The model under review builds one solid part; all positions refer to its coordinate system, in mm. Face numbers are marked on the shaded views. A direction names the side the tool comes from. Round coordinates to 2 decimals unless told otherwise and drop trailing zeros. Order: outer loops, then holes, each group sorted by start corner. A loop starts at its lowest first (then second) coordinate and runs counter-clockwise, first axis right, second up. Notation, with made-up numbers: M 55,47 L 89,47 A26 cw 89,84 Z; hole C -18,-19 d4. An arc over 180 degrees is marked long. One line per item, written item: value. Start each with the question number.
from build123d import *

# Parameters (mm, degrees)
SKETCH2_W           = 6.35
SKETCH2_H           = 2.3
BOSS_EXTRUDE1_DEPTH = 2
SKETCH4_W           = 9.35
SKETCH4_H           = 5.3
BOSS_EXTRUDE3_DEPTH = 2
FILLET1_R           = 1


with BuildPart() as part:
    # Sketch2 → Boss-Extrude1 (new body)
    with BuildSketch(Plane.XY):
        with Locations((-2.304595016, -0.87305296)):
            Rectangle(SKETCH2_W, SKETCH2_H)
    extrude(amount=BOSS_EXTRUDE1_DEPTH)

    # Sketch4 → Boss-Extrude3 (add)
    with BuildSketch(Plane.XY.offset(2)):
        with Locations((-2.304595016, -0.87305296)):
            Rectangle(SKETCH4_W, SKETCH4_H)
    extrude(amount=BOSS_EXTRUDE3_DEPTH)

    # Fillet1
    fillet1_edges = [part.edges().sort_by_distance(p)[0] for p in [
        (2.370404984, -0.87305296, 4),
        (-2.304595016, 1.77694704, 4),
        (-6.979595016, -0.87305296, 4),
        (-2.304595016, -3.52305296, 4),
    ]]
    fillet(fillet1_edges, radius=FILLET1_R)


solid = part.part
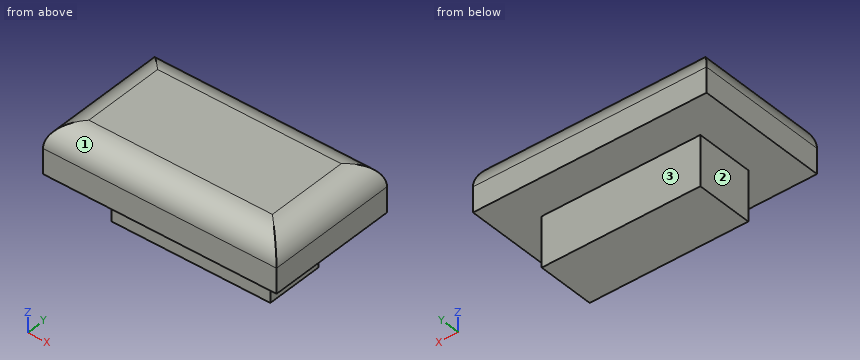
Item 1: Machinability: for the marked faces 1, 2 and 3, which of the approach directions +Z, -Z, +X, -X, +Y, -Y give a long, thin tool a straight path to every point of the face, cutting with its end or side? Answer none if there is none.
Item 2: Consider section A-A, the plane x = -1.5. Give the boundary of the cut face in (y, z).
Item 3: Consider section D-D, the plane y = -2.15. Give the boundary of the cut face in (x, z).
Item 4: Wall thickness on L1, parallel to Z at x = 0.75, y = -2.6; L2, parallel to X at y = -0.2, z = 0.85; L3, parallel to Y at x = -3, z = 1.2: over which ranges is each line inside the solid? List them lowest first.
Item 5: Consider section C-C, the plane z = 1.6. Give the boundary of the cut face in (x, y).
Item 6: Consider section B-B, the plane y = 0.05. Give the boundary of the cut face in (x, z), then the cut area to 3 significant figures.
Item 7: Clearance check with flat-ended pins moving along their axes: P1, Ø0.6, axis at x = -3.5, z = 1.5, coming from the -Y side; P2, Ø0.6, axis at y = -1, z = 1, coming from the -X side; P3, Ø1, axis at x = -2, z = 1, coming from the +Y side. State where each tip first meets the part, or that it passes through.
Computed:
1. face 1: +Z, +X, -X, -Y
1. face 2: -Z, -X, +Y, -Y
1. face 3: -Z, +X, -X, +Y
2. outline: M -3.52,2 L -2.02,2 L -2.02,0 L 0.28,0 L 0.28,2 L 1.78,2 L 1.78,3 A1 ccw 0.78,4 L -2.52,4 A1 ccw -3.52,3 Z
3. outline: M -6.98,2 L 2.37,2 L 2.37,3 A1 ccw 1.37,4 L -5.98,4 A1 ccw -6.98,3 Z
4. L1: z = 2 to 4
4. L2: x = -5.48 to 0.87
4. L3: y = -2.02 to 0.28
5. outline: M -5.48,-2.02 L 0.87,-2.02 L 0.87,0.28 L -5.48,0.28 Z
6. outline: M -6.98,2 L -5.48,2 L -5.48,0 L 0.87,0 L 0.87,2 L 2.37,2 L 2.37,3 A1 ccw 1.37,4 L -5.98,4 A1 ccw -6.98,3 Z
6. area: 31.0 mm^2
7. P1: stops at y = -2.02
7. P2: stops at x = -5.48
7. P3: stops at y = 0.28
